Autodesk Inventor part; units mm, degrees
ref_plane "Work Plane1" through (30.1625, 0, 0) normal (0, 0, -1) x (1, 0, 0)
ref_plane "YZ Plane" through (0, 0, 0) normal (1, 0, 0) x (0, 1, 0)
ref_plane "XZ Plane" through (0, 0, 0) normal (0, 1, 0) x (-1, 0, 0)
sketch "Эскиз1" plane through (0, 0, 0) normal (0, 0, 1) x (1, 0, 0)
  line L0 (-5, 0) -> (12, 0)
  line L1 (12, 0) -> (12, 4)
  line L2 (12, 4) -> (1.25, 4)
  line L3 (1.25, 4) -> (0.4832, 4)
  line L4 (0.4832, 4) -> (0, 4)
  line L5 (0, 4) -> (0, 6.5)
  line L6 (-8.4, 0) -> (15.4, 0)
  line L7 (0, -1.3) -> (0, 7.8)
  line L8 (-5, 0) -> (-5, 6.5)
  line L9 (0, 6.5) -> (-5, 6.5)
  dimension "d0" = 12
  dimension "d1" = 10.75
  dimension "d2" = 0.7668
  dimension "d3" = 5
  dimension "d4" = 8
  dimension "d5" = 8
  dimension "d9" = 13
  dimension "d10" = 0
revolve "Базовый элемент" add sketch "Эскиз1" angle 360 about axis through (-5, 0, 0) along (1, 0, 0)
sketch "Эскиз2" plane through (-5, 0, 0) normal (-1, 0, 0) x (0, 0, 1)
  circle A0 centre (0, 0) radius 6.5
  line L0 (0, 0) -> (0, 6.5)
  line L1 (-6.5, 0.875) -> (6.5, 0.875)
  line L2 (6.5, 0.875) -> (6.5, -0.875)
  line L3 (6.5, -0.875) -> (-6.5, -0.875)
  line L4 (-6.5, -0.875) -> (-6.5, 0.875)
  line L5 (-6.5, 0) -> (6.5, 0) construction
  line L6 (0, 0.875) -> (0, -0.875) construction
  dimension "d11" = 1.75
  dimension "d12" = 13
fillet "Сопряжение1" radius 0.01 1 edges at (-5, -6.5, 0)
extrude "Паз" cut sketch "Эскиз2" against normal blind 3.5 contours A0 L3 L1 | L2 L3 A0 | A0 L1 L2 | L3 L4 A0 | A0 L4 L1
thread "Резьба"
chamfer "Chamfer4" distance 0.8 angle 45 1 edges at (12, -4, 0)
ref_plane "Work Plane1" through (30.1625, 0, 0) normal (0, 0, -1) x (1, 0, 0)
equation "\"d11\" = SBR"
equation "\"d12\" = KOD"
equation "\"d13\" = RR"
equation "\"d16\" = STI"
equation "\"d14\" = GEL"
equation "\"d40\" = 0.1 * GD"
equation "\"d0\" = NLG"
equation "\"d1\" = GEL"
equation "\"d2\" = GAL"
equation "\"d3\" = KOH"
equation "\"d4\" = GD"
equation "\"d5\" = BDM"
equation "\"d9\" = KOD"
equation "\"GD\" = NND"
equation "\"NLG\" = 12"
equation "\"GEL\" = 10.75"
equation "\"KOD\" = 13"
equation "\"KOH\" = 5"
equation "\"GAL\" = 0.61345 * PTC"
equation "\"BDM\" = NND"
equation "\"RR\" = 0.01"
equation "\"SBR\" = 1.75"
equation "\"STI\" = 3.5"
equation "\"KEWI\" = 0"
equation "\"GUL\" = 0.61345 * PTC"
equation "\"SPD\" = NND - 1.2269 * PTC"
equation "\"PTC\" = 1.25"
equation "\"THREADDIA\" = 8"
equation "\"TOA\" = 30deg"
equation "\"FAWI\" = 45deg"
equation "\"NND\" = 8"
equation "\"GD1\" = THREADDIA - 1.2269 * PTC"
properties part number "Винт M8-6gx12 ГОСТ 1491-80" material "Сталь, мягкая"
Design review of the part built by this model. Coordinates are the model's own, in mm. A direction names the side the tool comes from. Give positions to 0.01 mm unless a question says otherwise; leave off trailing zeros. Loops run counter-clockwise (first coordinate to the right, second up) from the corner with the lowest first, then second, coordinate; pieces in that order, holes last. Notation, with made-up numbers: (83.25, 81.25) - (125.25, 81.25) arc R34 ccw to (125.25, 117.25) - close; hole circle Ø10 at (31, -29). An arc over 180 degrees is marked (long way). Use CSV: the item, a comma, the result in double quotes. Start each with the question number.
1. Add section D-D (x = 4.25). State the section outline as (y, z) points, plus the area to 3 significant figures.
2. Wall thickness on L1, parallel to X at y = 0.75, z = 4.25; L2, parallel to X at y = 6, z = 1.5; L3, parallel to Y at x = -2, z = -4.75 (3 decimals): over which ranges is each line inside the solid? List them lowest first.
3. Machinability: for faces 5 (the flat face through (-5, -3, 0)), 6 (the flat face through (0, 3, 3)), 7 (the flat face through (-3, -0.875, 0)), which of the approach directions +Z, -Z, +X, -X, +Y, -Y give a long, thin tool a straight path to every point of the face, cutting with its end or side? Answer none if there is none.
4. Add section C-C (z = 0). State the section outline as (x, y) points (3 decimals), plus the area to 3 significant figures.
5. Draft analysis for pull direction Y (two halves, no side actions). For faces 1 (the flat face through (-1.5, 0, 0)), 2 (the flat face through (-3, 0.875, 0)), 3 (the cylindrical face through (5.522, -0.867, 3.905)), 4 (the flat face through (12, 0, 0)), state which applies: released by +Y, released by -Y, zero draft, split by the parting line, or undercut.
6. Insertion check: P1, Ø2, axis at x = 0.5, z = -2.5, coming from the +Y side; P2, Ø4, axis at x = -4, z = -2.5, coming from the -Y side; P3, Ø4, axis at x = -1, z = -4, coming from the -Y side. Each pin has a flat end and moves straight along its axis. Give the tip position at first contact, or say it passes through.
7. Add section A-A (x = -2). State the section outline as (y, z) points (3 decimals).
8. Add section B-B (y = 0). State the section outline as (x, z) points.
Results found:
1,outline,"circle Ø8 at (0, 0)"
1,area,"50.3 mm²"
2,L1,"x = -1.5 to 0"
2,L2,"x = -5 to 0"
2,L3,"y = -4.437 to -0.875, 0.875 to 4.437"
3,face 5,"+Z, -Z, -X, +Y, -Y"
3,face 6,"+X"
3,face 7,"+Z, -Z, -X"
4,outline,"(-5, -6.49) arc R0.01 ccw to (-4.99, -6.5) - (0, -6.5) - (0, -4) - (11.2, -4) - (12, -3.2) - (12, 3.2) - (11.2, 4) - (0, 4) - (0, 6.5) - (-4.99, 6.5) arc R0.01 ccw to (-5, 6.49) - (-5, 0.875) - (-1.5, 0.875) - (-1.5, -0.875) - (-5, -0.875) - close"
4,area,"154 mm²"
5,face 1,"undercut"
5,face 2,"undercut"
5,face 3,"split by the parting line"
5,face 4,"zero draft"
6,P1,"stops at y = 6.29"
6,P2,"stops at y = -6.48"
6,P3,"stops at y = -6.18"
7,outline,"(-0.875, -6.441) - (-0.875, 6.441) arc R6.5 ccw to start; (0.875, -6.441) arc R6.5 ccw to (0.875, 6.441) - close"
8,outline,"(-1.5, -6.5) - (0, -6.5) - (0, -4) - (11.2, -4) - (12, -3.2) - (12, 3.2) - (11.2, 4) - (0, 4) - (0, 6.5) - (-1.5, 6.5) - close"
